Can you work these out from the model? Positions are in its coordinate system, mm. Give positions to 0.01 mm unless a question says otherwise; leave off trailing zeros. Loops run counter-clockwise (first coordinate to the right, second up) from the corner with the lowest first, then second, coordinate; pieces in that order, holes last. Notation, with made-up numbers: (24, 57) - (69, 57) arc R25 ccw to (69, 69) - close; hole circle Ø4 at (84, 54.25). An arc over 180 degrees is marked (long way). Use a Markdown table: item, result. Add a question column.
```python
from build123d import *

# Parameters (mm, degrees)
SKETCH1_W           = 137.24989985
SKETCH1_H           = 79.804399954
SKETCH1_R           = 0.750000024
SKETCH1_R_2         = 1.000000032
SKETCH1_R_3         = 1.750000056
SKETCH1_R_4         = 3.249999977
BOSS_EXTRUDE1_DEPTH = 0.8382
SKETCH2_W           = 7.62
SKETCH2_H           = 0.8382
BOSS_EXTRUDE2_DEPTH = 5.08


with BuildPart() as part:
    # Sketch1 → Boss-Extrude1 (new body)
    with BuildSketch(Plane(origin=(0, 0, 0), x_dir=(1, 0, 0), z_dir=(0, 1, 0))):
        with Locations((68.624949925, 39.902199977)):
            Rectangle(SKETCH1_W, SKETCH1_H)
        with Locations(Location((2.859372911, 10.000000066, 0), (0, 0, 270))):
            Circle(SKETCH1_R, mode=Mode.SUBTRACT)
        with Locations(Location((8.578106711, 10.000000066, 0), (0, 0, 270))):
            Circle(SKETCH1_R, mode=Mode.SUBTRACT)
        with Locations(Location((14.296840511, 10.000000066, 0), (0, 0, 270))):
            Circle(SKETCH1_R, mode=Mode.SUBTRACT)
        with Locations(Location((20.015574311, 10.000000066, 0), (0, 0, 270))):
            Circle(SKETCH1_R, mode=Mode.SUBTRACT)
        with Locations(Location((25.734308111, 10.000000066, 0), (0, 0, 270))):
            Circle(SKETCH1_R, mode=Mode.SUBTRACT)
        with Locations(Location((31.453041911, 10.000000066, 0), (0, 0, 270))):
            Circle(SKETCH1_R, mode=Mode.SUBTRACT)
        with Locations(Location((37.171775711, 10.000000066, 0), (0, 0, 270))):
            Circle(SKETCH1_R, mode=Mode.SUBTRACT)
        with Locations(Location((42.890509511, 10.000000066, 0), (0, 0, 270))):
            Circle(SKETCH1_R, mode=Mode.SUBTRACT)
        with Locations(Location((48.609243311, 10.000000066, 0), (0, 0, 270))):
            Circle(SKETCH1_R, mode=Mode.SUBTRACT)
        with Locations(Location((54.327977111, 10.000000066, 0), (0, 0, 270))):
            Circle(SKETCH1_R, mode=Mode.SUBTRACT)
        with Locations(Location((60.046710911, 10.000000066, 0), (0, 0, 270))):
            Circle(SKETCH1_R, mode=Mode.SUBTRACT)
        with Locations(Location((65.765444711, 10.000000066, 0), (0, 0, 270))):
            Circle(SKETCH1_R, mode=Mode.SUBTRACT)
        with Locations(Location((71.484178511, 10.000000066, 0), (0, 0, 270))):
            Circle(SKETCH1_R, mode=Mode.SUBTRACT)
        with Locations(Location((77.202912311, 10.000000066, 0), (0, 0, 270))):
            Circle(SKETCH1_R, mode=Mode.SUBTRACT)
        with Locations(Location((82.921646111, 10.000000066, 0), (0, 0, 270))):
            Circle(SKETCH1_R, mode=Mode.SUBTRACT)
        with Locations(Location((88.640379911, 10.000000066, 0), (0, 0, 270))):
            Circle(SKETCH1_R, mode=Mode.SUBTRACT)
        with Locations(Location((94.359113711, 10.000000066, 0), (0, 0, 270))):
            Circle(SKETCH1_R, mode=Mode.SUBTRACT)
        with Locations(Location((100.077847511, 10.000000066, 0), (0, 0, 270))):
            Circle(SKETCH1_R, mode=Mode.SUBTRACT)
        with Locations(Location((105.796581311, 10.000000066, 0), (0, 0, 270))):
            Circle(SKETCH1_R, mode=Mode.SUBTRACT)
        with Locations(Location((111.515315111, 10.000000066, 0), (0, 0, 270))):
            Circle(SKETCH1_R, mode=Mode.SUBTRACT)
        with Locations(Location((117.234048911, 10.000000066, 0), (0, 0, 270))):
            Circle(SKETCH1_R, mode=Mode.SUBTRACT)
        with Locations(Location((122.952782711, 10.000000066, 0), (0, 0, 270))):
            Circle(SKETCH1_R, mode=Mode.SUBTRACT)
        with Locations(Location((128.671516511, 10.000000066, 0), (0, 0, 270))):
            Circle(SKETCH1_R, mode=Mode.SUBTRACT)
        with Locations(Location((134.390250311, 10.000000066, 0), (0, 0, 270))):
            Circle(SKETCH1_R, mode=Mode.SUBTRACT)
        with Locations(Location((2.859372911, 17.000000036, 0), (0, 0, 270))):
            Circle(SKETCH1_R_2, mode=Mode.SUBTRACT)
        with Locations(Location((14.296865911, 17.000000036, 0), (0, 0, 270))):
            Circle(SKETCH1_R_2, mode=Mode.SUBTRACT)
        with Locations(Location((25.734358911, 17.000000036, 0), (0, 0, 270))):
            Circle(SKETCH1_R_2, mode=Mode.SUBTRACT)
        with Locations(Location((37.171851911, 17.000000036, 0), (0, 0, 270))):
            Circle(SKETCH1_R_2, mode=Mode.SUBTRACT)
        with Locations(Location((48.609344911, 17.000000036, 0), (0, 0, 270))):
            Circle(SKETCH1_R_2, mode=Mode.SUBTRACT)
        with Locations(Location((60.046837911, 17.000000036, 0), (0, 0, 270))):
            Circle(SKETCH1_R_2, mode=Mode.SUBTRACT)
        with Locations(Location((71.484330911, 17.000000036, 0), (0, 0, 270))):
            Circle(SKETCH1_R_2, mode=Mode.SUBTRACT)
        with Locations(Location((82.921823911, 17.000000036, 0), (0, 0, 270))):
            Circle(SKETCH1_R_2, mode=Mode.SUBTRACT)
        with Locations(Location((94.359316911, 17.000000036, 0), (0, 0, 270))):
            Circle(SKETCH1_R_2, mode=Mode.SUBTRACT)
        with Locations(Location((105.796809911, 17.000000036, 0), (0, 0, 270))):
            Circle(SKETCH1_R_2, mode=Mode.SUBTRACT)
        with Locations(Location((117.234302911, 17.000000036, 0), (0, 0, 270))):
            Circle(SKETCH1_R_2, mode=Mode.SUBTRACT)
        with Locations(Location((128.671795911, 17.000000036, 0), (0, 0, 270))):
            Circle(SKETCH1_R_2, mode=Mode.SUBTRACT)
        with Locations(Location((7.52228568, 36.999999914, 0), (0, 0, 270))):
            Circle(SKETCH1_R_3, mode=Mode.SUBTRACT)
        with Locations(Location((18.959777325, 36.999999914, 0), (0, 0, 270))):
            Circle(SKETCH1_R_3, mode=Mode.SUBTRACT)
        with Locations(Location((30.397268971, 36.999999914, 0), (0, 0, 270))):
            Circle(SKETCH1_R_3, mode=Mode.SUBTRACT)
        with Locations(Location((41.834760616, 36.999999914, 0), (0, 0, 270))):
            Circle(SKETCH1_R_3, mode=Mode.SUBTRACT)
        with Locations(Location((53.272252261, 36.999999914, 0), (0, 0, 270))):
            Circle(SKETCH1_R_3, mode=Mode.SUBTRACT)
        with Locations(Location((64.709743907, 36.999999914, 0), (0, 0, 270))):
            Circle(SKETCH1_R_3, mode=Mode.SUBTRACT)
        with Locations(Location((76.147235552, 36.999999914, 0), (0, 0, 270))):
            Circle(SKETCH1_R_3, mode=Mode.SUBTRACT)
        with Locations(Location((87.584727197, 36.999999914, 0), (0, 0, 270))):
            Circle(SKETCH1_R_3, mode=Mode.SUBTRACT)
        with Locations(Location((99.022218843, 36.999999914, 0), (0, 0, 270))):
            Circle(SKETCH1_R_3, mode=Mode.SUBTRACT)
        with Locations(Location((110.459710488, 36.999999914, 0), (0, 0, 270))):
            Circle(SKETCH1_R_3, mode=Mode.SUBTRACT)
        with Locations(Location((121.897202133, 36.999999914, 0), (0, 0, 270))):
            Circle(SKETCH1_R_3, mode=Mode.SUBTRACT)
        with Locations(Location((133.334693779, 36.999999914, 0), (0, 0, 270))):
            Circle(SKETCH1_R_3, mode=Mode.SUBTRACT)
        with Locations(Location((5.033610572, 43.999999884, 0), (0, 0, 270))):
            Circle(SKETCH1_R_4, mode=Mode.SUBTRACT)
        with Locations(Location((16.471103572, 43.999999884, 0), (0, 0, 270))):
            Circle(SKETCH1_R_4, mode=Mode.SUBTRACT)
        with Locations(Location((27.908596572, 43.999999884, 0), (0, 0, 270))):
            Circle(SKETCH1_R_4, mode=Mode.SUBTRACT)
        with Locations(Location((39.346089572, 43.999999884, 0), (0, 0, 270))):
            Circle(SKETCH1_R_4, mode=Mode.SUBTRACT)
        with Locations(Location((50.783582572, 43.999999884, 0), (0, 0, 270))):
            Circle(SKETCH1_R_4, mode=Mode.SUBTRACT)
        with Locations(Location((62.221075572, 43.999999884, 0), (0, 0, 270))):
            Circle(SKETCH1_R_4, mode=Mode.SUBTRACT)
        with Locations(Location((73.658568572, 43.999999884, 0), (0, 0, 270))):
            Circle(SKETCH1_R_4, mode=Mode.SUBTRACT)
        with Locations(Location((85.096061572, 43.999999884, 0), (0, 0, 270))):
            Circle(SKETCH1_R_4, mode=Mode.SUBTRACT)
        with Locations(Location((96.533554572, 43.999999884, 0), (0, 0, 270))):
            Circle(SKETCH1_R_4, mode=Mode.SUBTRACT)
        with Locations(Location((107.971047572, 43.999999884, 0), (0, 0, 270))):
            Circle(SKETCH1_R_4, mode=Mode.SUBTRACT)
        with Locations(Location((119.408540572, 43.999999884, 0), (0, 0, 270))):
            Circle(SKETCH1_R_4, mode=Mode.SUBTRACT)
        with Locations(Location((130.846033572, 43.999999884, 0), (0, 0, 270))):
            Circle(SKETCH1_R_4, mode=Mode.SUBTRACT)
        with Locations(Location((2.859372911, 62.999999984, 0), (0, 0, 270))):
            Circle(SKETCH1_R_2, mode=Mode.SUBTRACT)
        with Locations(Location((14.296865911, 62.999999984, 0), (0, 0, 270))):
            Circle(SKETCH1_R_2, mode=Mode.SUBTRACT)
        with Locations(Location((25.734358911, 62.999999984, 0), (0, 0, 270))):
            Circle(SKETCH1_R_2, mode=Mode.SUBTRACT)
        with Locations(Location((37.171851911, 62.999999984, 0), (0, 0, 270))):
            Circle(SKETCH1_R_2, mode=Mode.SUBTRACT)
        with Locations(Location((48.609344911, 62.999999984, 0), (0, 0, 270))):
            Circle(SKETCH1_R_2, mode=Mode.SUBTRACT)
        with Locations(Location((60.046837911, 62.999999984, 0), (0, 0, 270))):
            Circle(SKETCH1_R_2, mode=Mode.SUBTRACT)
        with Locations(Location((71.484330911, 62.999999984, 0), (0, 0, 270))):
            Circle(SKETCH1_R_2, mode=Mode.SUBTRACT)
        with Locations(Location((82.921823911, 62.999999984, 0), (0, 0, 270))):
            Circle(SKETCH1_R_2, mode=Mode.SUBTRACT)
        with Locations(Location((94.359316911, 62.999999984, 0), (0, 0, 270))):
            Circle(SKETCH1_R_2, mode=Mode.SUBTRACT)
        with Locations(Location((105.796809911, 62.999999984, 0), (0, 0, 270))):
            Circle(SKETCH1_R_2, mode=Mode.SUBTRACT)
        with Locations(Location((117.234302911, 62.999999984, 0), (0, 0, 270))):
            Circle(SKETCH1_R_2, mode=Mode.SUBTRACT)
        with Locations(Location((128.671795911, 62.999999984, 0), (0, 0, 270))):
            Circle(SKETCH1_R_2, mode=Mode.SUBTRACT)
    extrude(amount=BOSS_EXTRUDE1_DEPTH)

    # Sketch2 → Boss-Extrude2 (add)
    with BuildSketch(Plane.ZY):
        with Locations((-75.994399954, 0.4191)):
            Rectangle(SKETCH2_W, SKETCH2_H)
        with Locations((-3.81, 0.4191)):
            Rectangle(SKETCH2_W, SKETCH2_H)
    extrude(amount=BOSS_EXTRUDE2_DEPTH)


solid = part.part
```
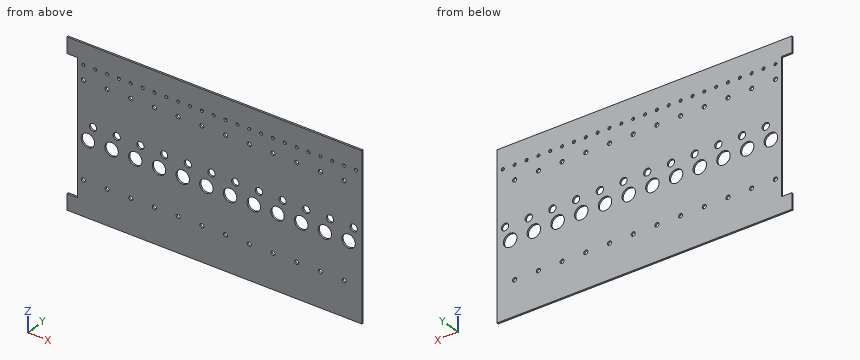
1. Suppose I cut it at A-A (z = -44). State how many separate pieces and enclosed holes the cut face has, and give its area (3 significant figures).
2. Will this pin go through, and if not, where does the flat tip stop? P1, Ø1.8, axis at x = 60.05, z = -17, coming from the -Y side.
3. Please list where these lines run through material, in increasing order: line 1 along Z through (x, y) = (41, 0.45); line 2 along Z through (x, y) = (128, 0.55); line 3 along Z through (x, y) = (100, 0.6). Write a range as [from, to].
4. Suppose I cut it at B-B (z = -12.5). List the corners of the cut face in (x, y) for me, and give its area (3 significant figures).
Results below:
| question | item | result |
|---|---|---|
| 1 | separate pieces | 13 |
| 1 | enclosed holes | 0 |
| 1 | area | 49.7 mm² |
| 2 | P1 | through |
| 3 | line 1 | [-79.8, -46.8], [-41.2, -38.54], [-35.46, 0] |
| 3 | line 2 | [-79.8, -63.74], [-62.26, -45.57], [-42.43, -17.74], [-16.26, -10.33], [-9.67, 0] |
| 3 | line 3 | [-79.8, -38.45], [-35.55, -10.75], [-9.25, 0] |
| 4 | outline | (0, 0) - (137.25, 0) - (137.25, 0.84) - (0, 0.84) - close |
| 4 | area | 115 mm² |
